Print and shaded views of the part. All mm, measured from the part's lowest x, y and z. A direction names the side the tool comes from. Give positions to 0.01 mm unless a question says otherwise; leave off trailing zeros. Loops run counter-clockwise (first coordinate to the right, second up) from the corner with the lowest first, then second, coordinate; pieces in that order, holes last.
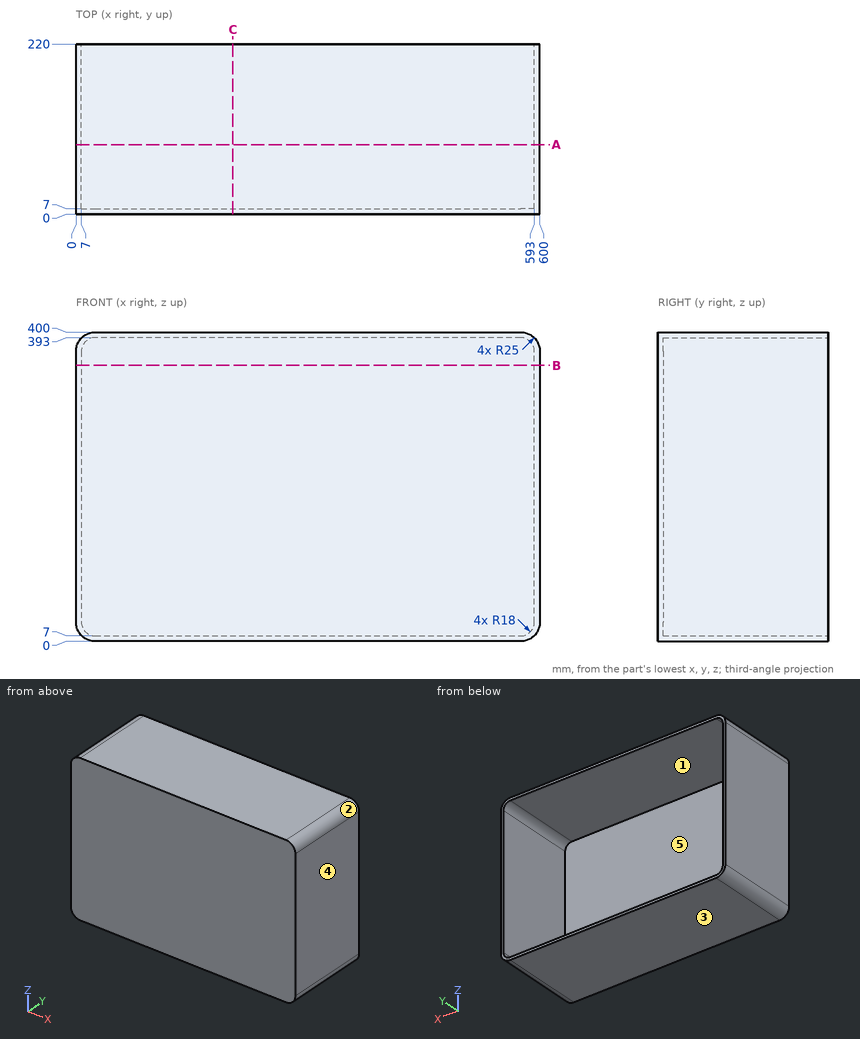
1. Saw through at C-C, the plane x = 203. List the corners of the cut face in (y, z), and give its area (3 significant figures).
Responses:
outline: (0, 0) - (220, 0) - (220, 7) - (7, 7) - (7, 393) - (220, 393) - (220, 400) - (0, 400) - close
area: 5,780 mm2
2. Pull direction Z, two halves, no side cores. Call the marked faces 1, 2 and 3: released by +Z, released by -Z, zero draft, split by the parting line, or undercut.
Responses:
face 1: undercut
face 2: released by +Z
face 3: released by -Z
3. Drop a flat-ended pin along its axis: pin 1 (1.5 mm diameter, centred on x = 462, z = 148.5, fed in from +Y). Give the stop position or say it passes through.
Responses:
pin 1: stops at y = 7
4. Saw through at A-A, the plane y = 90. List the corners of the cut face in (x, z).
Responses:
outline: (0, 25) arc R25 ccw to (25, 0) - (575, 0) arc R25 ccw to (600, 25) - (600, 375) arc R25 ccw to (575, 400) - (25, 400) arc R25 ccw to (0, 375) - close; hole (7, 25) arc R18 ccw to (25, 7) - (575, 7) arc R18 ccw to (593, 25) - (593, 375) arc R18 ccw to (575, 393) - (25, 393) arc R18 ccw to (7, 375) - close
5. Saw through at B-B, the plane z = 357. List the corners of the cut face in (x, y).
Responses:
outline: (0, 0) - (600, 0) - (600, 220) - (593, 220) - (593, 7) - (7, 7) - (7, 220) - (0, 220) - close
6. Probe line 1 along Z through (x, y) = (166.5, 12); line 2 along X through (y, z) = (167, 244); line 3 along Y through (x, z) = (458, 358). List the from-to ranges inside material, lowest first.
Responses:
line 1: z = 0 to 7, 393 to 400
line 2: x = 0 to 7, 593 to 600
line 3: y = 0 to 7
7. Tool access for the marked faces 4 and 5: list every direction of +Z, -Z, +X, -X, +Y, -Y with a clear straight run to the whole face (end or side of a thin tool).
Responses:
face 4: +Z, -Z, +X, +Y, -Y
face 5: +Y
